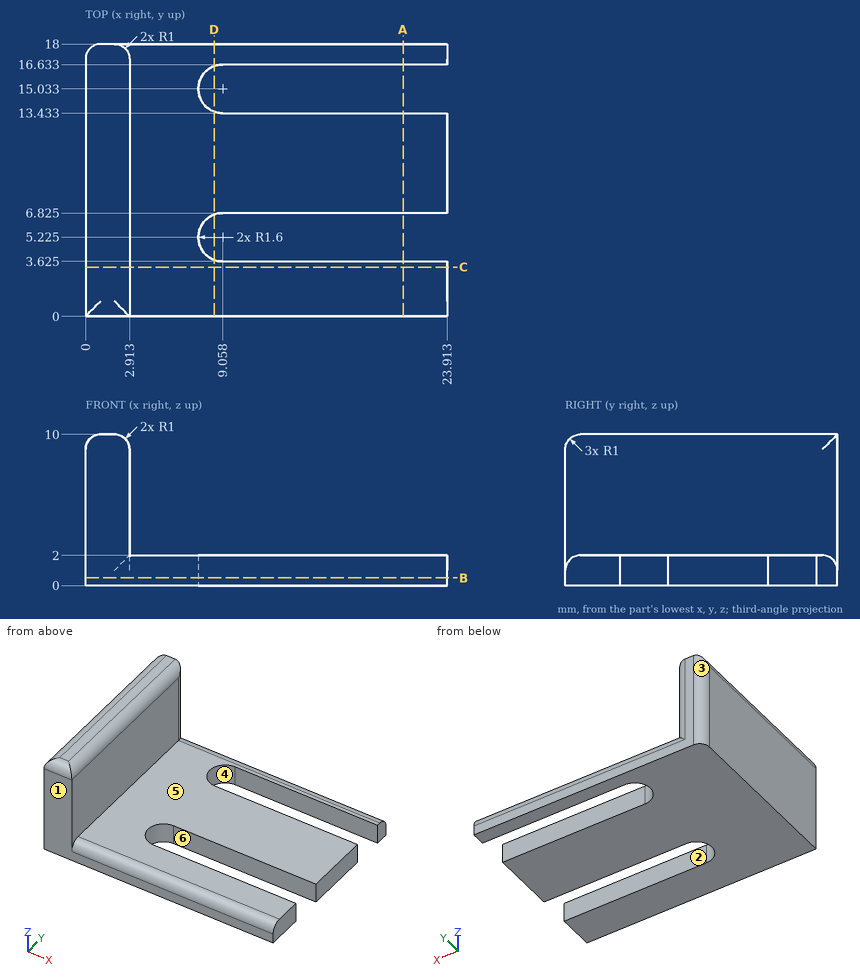
The drawing under review shows one solid part. Ordinate dimensions are in mm from its lowest x, y, z. A direction names the side the tool comes from. Coordinates: 2 decimals unless noted, no trailing zeros. Write each loop counter-clockwise with the first axis right and the second up, starting at its lowest first coordinate (ties: lowest second). Pieces come first, ordered by that corner, then holes.
1) Mouldability with a two-part tool opening along Y and no side actions: class the marked faces 3, 4, 5 and 6 as +Y half, -Y half, draft (parallel to the pull), parting line (faces both ways), or undercut.
2) Machinability: for the marked faces 1 and 2, which of the approach directions +Z, -Z, +X, -X, +Y, -Y give a long, thin tool a straight path to every point of the face, cutting with its end or side? Answer none if there is none.
3) Add section C-C (y = 3.25). Write out the cut boundary in (x, z).
4) Add section B-B (z = 0.5). Write out the cut boundary in (x, y) (1 decimal), plus the area to 3 significant figures.
5) To check wall thickness, follow L1, parallel to Z at x = 10.75, y = 10.5; L2, parallel to X at y = 15.25, z = 5.75; L3, parallel to Y at x = 18, z = 1.5 (1 decimal). State the ranges of each line that lie inside material, in increasing order.
6) Insertion check: pin 1 (1 mm diameter, centred on x = 19, y = 2, fed in from +Z); pin 2 (4 mm diameter, centred on x = 12, z = 3.5, fed in from +Y) (1 decimal); pin 3 (5 mm diameter, centred on y = 9, z = 5, fed in from +X). Each pin has a flat end and moves straight along its axis. Give the tip position at first contact, or say it passes through.
7) Add section A-A (x = 21). State how many separate pieces and enclosed holes the cut face has.
8) Add section D-D (x = 8.5). Write out the cut boundary in (y, z) (1 decimal).
Check result:
1. face 3: +Y half
1. face 4: undercut
1. face 5: draft
1. face 6: undercut
2. face 1: +Z, -Z, +X, -X, -Y
2. face 2: +Z, -Z, +X
3. outline: (0, 0) - (23.91, 0) - (23.91, 2) - (2.91, 2) - (2.91, 9) arc R1 ccw to (1.91, 10) - (1, 10) arc R1 ccw to (0, 9) - close
4. outline: (0, 0) - (23.9, 0) - (23.9, 3.6) - (9.1, 3.6) arc R1.6 cw to (9.1, 6.8) - (23.9, 6.8) - (23.9, 13.4) - (9.1, 13.4) arc R1.6 cw to (9.1, 16.6) - (23.9, 16.6) - (23.9, 18) - (1, 18) arc R1 ccw to (0, 17) - close
4. area: 327 mm2
5. L1: z = 0 to 2
5. L2: x = 0 to 2.91
5. L3: y = 0.1 to 3.6, 6.8 to 13.4, 16.6 to 17.9
6. pin 1: stops at z = 2
6. pin 2: stops at y = 17.9
6. pin 3: stops at x = 2.91
7. separate pieces: 3
7. enclosed holes: 0
8. outline: (0, 0) - (3.7, 0) - (3.7, 2) - (1, 2) arc R1 ccw to (0, 1) - close; (6.7, 0) - (13.5, 0) - (13.5, 2) - (6.7, 2) - close; (16.5, 0) - (18, 0) - (18, 1) arc R1 ccw to (17, 2) - (16.5, 2) - close
